Input: dimensioned drawing with shaded views. Units: mm. Origin: part minimum x, y, z. Round coordinates to 2 decimals unless told otherwise and drop trailing zeros. Loops run counter-clockwise (first coordinate to the right, second up) from the corner with the lowest first, then second, coordinate; pieces in that order, holes last. Notation, with made-up numbers: M 1,18 L 30,18 A21 ccw 30,55 Z; hole C 59,2.25 d4. An arc over 180 degrees is marked long. Answer as a JSON object with one key per item and string values.
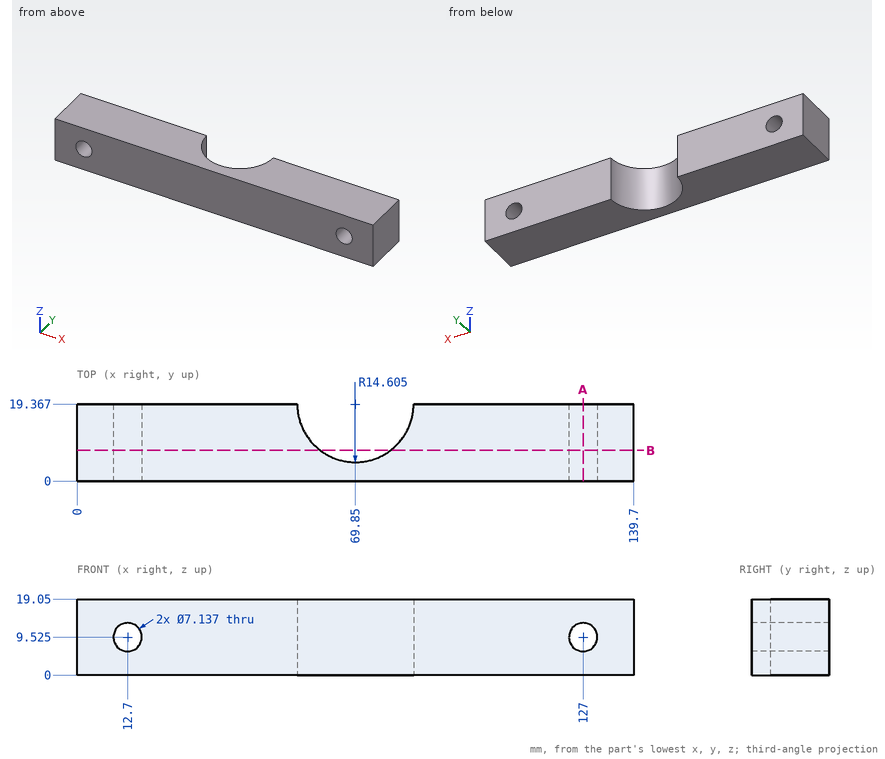
Item 1: Section B-B on y = 7.75. Give the number of separate pieces and of enclosed holes in the cut face, then the cut area to 3 significant figures.
Answer sheet:
{"separate pieces": "2", "enclosed holes": "2", "area": "2,240 mm²"}
Item 2: Section A-A on x = 127. Return the cut outline in (y, z).
Answer sheet:
{"outline": "M 0,0 L 19.37,0 L 19.37,5.96 L 0,5.96 Z; M 0,13.09 L 19.37,13.09 L 19.37,19.05 L 0,19.05 Z"}
Item 3: Line query: probe 1 along Z at (x, y) = (12.7, 4.75); probe 2 along X at (y, z) = (12.25, 12.75) (1 decimal); probe 3 along X at (y, z) = (18.5, 3.25). Output: solid intervals per line, ascending. Write a range as from..to.
Answer sheet:
{"probe 1": "z = 0..5.96, 13.09..19.05", "probe 2": "x = 0..11.2, 14.2..57.1, 82.6..125.5, 128.5..139.7", "probe 3": "x = 0..55.27, 84.43..139.7"}
Item 4: Contact query for flat-ended pins moving along their axis: pin 1 Ø1 at (x, z) = (67, 9.5) entering from +Y; pin 2 Ø6.5 at (x, z) = (12.7, 9.525) entering from -Y. Output: stop coordinate, or through.
Answer sheet:
{"pin 1": "stops at y = 5.15", "pin 2": "passes through"}
